Could you check a few things on this model? Use its own coordinates, in mm. Face numbers are marked on the shaded views. A direction names the side the tool comes from. Round coordinates to 2 decimals unless told otherwise and drop trailing zeros. Loops run counter-clockwise (first coordinate to the right, second up) from the corner with the lowest first, then second, coordinate; pieces in that order, holes last. Notation, with made-up numbers: (1, 39) -> (5, 39) arc R31 cw to (5, 68) -> close; hole circle Ø7 at (-29.5, 66). An arc over 180 degrees is marked (long way). Write each question's results on one line, items separated by ' | '.
from build123d import *

# Parameters (mm, degrees)
SKETCH1_R           = 80
BOSS_EXTRUDE1_DEPTH = 30
SKETCH2_R           = 17.5
CUT_EXTRUDE1_DEPTH  = 118.046999107
SKETCH3_R           = 10
CUT_EXTRUDE2_DEPTH  = 18.43204
CIRPATTERN1_START   = 11.567959846
CIRPATTERN1_DEPTH   = 18.432040154


# Read off the part's stored shape, not the designer's step: CirPattern1
with BuildPart() as part:
    # Sketch1 → Boss-Extrude1 (new body)
    with BuildSketch(Plane(origin=(0, 0, 0), x_dir=(1, 0, 0), z_dir=(0, 1, 0))):
        with Locations(Location((0, 0, 0), (0, 0, 270))):
            Circle(SKETCH1_R)
    extrude(amount=BOSS_EXTRUDE1_DEPTH)

    # Sketch2 → Cut-Extrude1 (cut, through all)
    with BuildSketch(Plane(origin=(0, 0, 0), x_dir=(1, 0, 0), z_dir=(0, 1, 0))):
        with Locations(Location((0, 0, 0), (0, 0, 270))):
            Circle(SKETCH2_R)
    extrude(amount=CUT_EXTRUDE1_DEPTH, mode=Mode.SUBTRACT)

    # Sketch3 → Cut-Extrude2 (cut)
    with BuildSketch(Plane(origin=(0, 30, 0), x_dir=(1, 0, 0), z_dir=(0, 1, 0))):
        with Locations((-23.230150503, 0)):
            Circle(SKETCH3_R)
    extrude(amount=-CUT_EXTRUDE2_DEPTH, mode=Mode.SUBTRACT)

    # CirPattern1 outline → CirPattern1 (cut)
    with BuildSketch(Plane(origin=(0, 0, 0), x_dir=(1, 0, 0), z_dir=(0, 1, 0)).offset(CIRPATTERN1_START)):
        with BuildLine():
            ThreePointArc((-16.054349116, -6.964759468), (-19.719877369, -9.3636522), (-24.059054546, -9.96558669))
            ThreePointArc((-24.059054546, -9.96558669), (-23.497264761, -23.497264761), (-9.965586691, -24.059054546))
            ThreePointArc((-9.965586691, -24.059054546), (0, -33.230150503), (9.965586691, -24.059054546))
            ThreePointArc((9.965586691, -24.059054546), (23.497264761, -23.497264761), (24.059054546, -9.965586691))
            ThreePointArc((24.059054546, -9.965586691), (33.230150503, 0), (24.059054546, 9.965586691))
            ThreePointArc((24.059054546, 9.965586691), (23.497264761, 23.497264761), (9.965586691, 24.059054546))
            ThreePointArc((9.965586691, 24.059054546), (0, 33.230150503), (-9.965586691, 24.059054546))
            ThreePointArc((-9.965586691, 24.059054546), (-23.497264761, 23.497264761), (-24.059054546, 9.965586691))
            ThreePointArc((-24.059054546, 9.965586691), (-19.719877369, 9.3636522), (-16.054349116, 6.964759468))
            ThreePointArc((-16.054349116, 6.964759468), (17.5, 0), (-16.054349116, -6.964759468))
        make_face()
    extrude(amount=CIRPATTERN1_DEPTH, mode=Mode.SUBTRACT)


solid = part.part
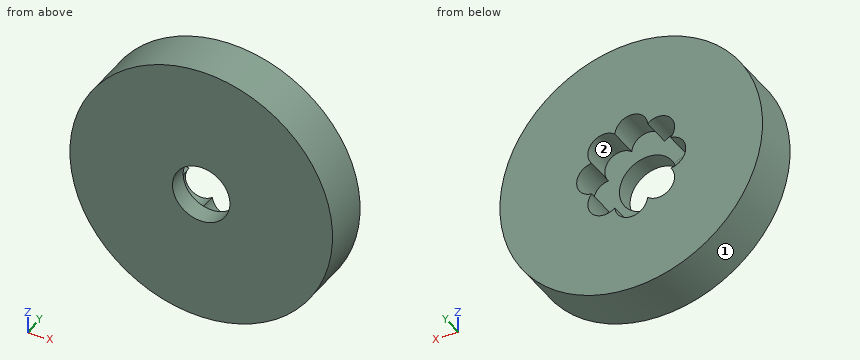
1) I want a section at D-D, the plane x = 44. Write out the boundary of the cut face in (y, z).
Model answer:
outline: (0, -66.81) -> (30, -66.81) -> (30, 66.81) -> (0, 66.81) -> close
2) I need wall thicknesses on line 1 (X direction, y = 8.5, z = 0); line 2 (Y direction, x = 2, z = -26.5); line 3 (X direction, y = 13.5, z = 9). Which ranges of each line are inside material? Lowest first, please.
Model answer:
line 1: x = -80 to -17.5, 17.5 to 80 | line 2: y = 0 to 11.57 | line 3: x = -79.49 to -27.59, 27.59 to 79.49
3) I want a section at B-B, the plane x = 0. Write out the boundary of the cut face in (y, z).
Model answer:
outline: (0, -80) -> (30, -80) -> (30, -33.23) -> (11.57, -33.23) -> (11.57, -17.5) -> (0, -17.5) -> close; (0, 17.5) -> (11.57, 17.5) -> (11.57, 33.23) -> (30, 33.23) -> (30, 80) -> (0, 80) -> close
4) I want a section at C-C, the plane y = 14. Write out the boundary of the cut face in (x, z).
Model answer:
outline: circle Ø160 at (0, 0); hole (-24.06, -9.97) arc R10 ccw to (-9.97, -24.06) arc R10 ccw to (9.97, -24.06) arc R10 ccw to (24.06, -9.97) arc R10 ccw to (24.06, 9.97) arc R10 ccw to (9.97, 24.06) arc R10 ccw to (-9.97, 24.06) arc R10 ccw to (-24.06, 9.97) arc R10 ccw to start
5) For the marked faces 1 and 2, which set-ups out of +Z, -Z, +X, -X, +Y, -Y let a thin tool reach every point of the face, with its end or its side?
Model answer:
face 1: +Y, -Y | face 2: +Y
6) I want a section at A-A, the plane z = 0. Write out the boundary of the cut face in (x, y).
Model answer:
outline: (-80, 0) -> (-17.5, 0) -> (-17.5, 11.57) -> (-33.23, 11.57) -> (-33.23, 30) -> (-80, 30) -> close; (17.5, 0) -> (80, 0) -> (80, 30) -> (33.23, 30) -> (33.23, 11.57) -> (17.5, 11.57) -> close
7) I'm going to push flat-ended pins straight in: pin 1 (6 mm diameter, centred on x = 15, y = 18, fed in from +Z); pin 2 (12 mm diameter, centred on y = 19.5, z = 30, fed in from +X); pin 3 (6 mm diameter, centred on y = 9.5, z = -45.5, fed in from +X). Where does each tip first touch, or does it pass through?
Model answer:
pin 1: stops at z = 79.09 | pin 2: stops at x = 76.32 | pin 3: stops at x = 67.78
